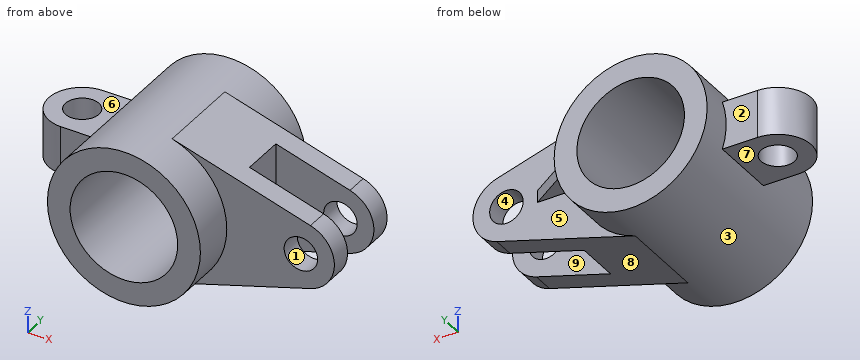
from build123d import *

# Parameters (mm, degrees)
SKETCH_1_R               = 32
SKETCH_1_R_2             = 22.5
EXTRUDE_1_DEPTH          = 72
SKETCH_2_R               = 7
EXTRUDE_2_DEPTH          = 36
CUT_EXTRUDE_1_DEPTH      = 9
EXTRUDE_3_DEPTH          = 14
SKETCH_5_R               = 7
CUT_EXTRUDE_2_DEPTH      = 33
CUT_EXTRUDE_2_DEPTH_BACK = 33
CUT_EXTRUDE_3_DEPTH      = 23
CUT_EXTRUDE_3_DEPTH_BACK = 43
EXTRUDE_4_DEPTH          = 2.5


with BuildPart() as part:
    # 草图1 → 凸台-拉伸1 (new body)
    with BuildSketch(Plane(origin=(0, 0, 0), x_dir=(1, 0, 0), z_dir=(0, 1, 0))):
        Circle(SKETCH_1_R)
        Circle(SKETCH_1_R_2, mode=Mode.SUBTRACT)
    extrude(amount=EXTRUDE_1_DEPTH)

    # 草图2 → 凸台-拉伸2 (add)
    with BuildSketch(Plane(origin=(0, 18, 0), x_dir=(1, 0, 0), z_dir=(0, 1, 0))):
        with BuildLine():
            Line((9.142857143, 30.66607512), (67, 13.416407865))
            ThreePointArc((67, 13.416407865), (77, 0), (67, -13.416407865))
            Line((67, -13.416407865), (9.142857143, -30.66607512))
            ThreePointArc((9.142857143, -30.66607512), (32, 0), (9.142857143, 30.66607512))
        make_face()
        with Locations((63, 0)):
            Circle(SKETCH_2_R, mode=Mode.SUBTRACT)
    extrude(amount=EXTRUDE_2_DEPTH)

    # 草图3 → 切除-拉伸1 (cut, symmetric)
    with BuildSketch(Plane(origin=(0, 36, 0), x_dir=(1, 0, 0), z_dir=(0, 1, 0))):
        with BuildLine():
            Line((36, 22.658822172), (36, -22.658822172))
            Line((36, -22.658822172), (67, -13.416407865))
            ThreePointArc((67, -13.416407865), (77, 0), (67, 13.416407865))
            Line((67, 13.416407865), (36, 22.658822172))
        make_face()
    extrude(amount=CUT_EXTRUDE_1_DEPTH, both=True, mode=Mode.SUBTRACT)

    # 草图4 → 凸台-拉伸3 (add, symmetric)
    with BuildSketch(Plane(origin=(0, 45, 0), x_dir=(1, 0, 0), z_dir=(0, 1, 0))):
        with BuildLine():
            Line((-30.330505487, 10), (-45, 10))
            Line((-45, 10), (-59, 10))
            Line((-59, 10), (-59, -10))
            Line((-59, -10), (-45, -10))
            Line((-45, -10), (-30.330505487, -10))
            ThreePointArc((-30.330505487, -10), (-31.936492655, 0), (-30.330505487, 10))
        make_face()
    extrude(amount=EXTRUDE_3_DEPTH, both=True)

    # 草图5 → 切除-拉伸2 (cut, two sides)
    with BuildSketch(Plane.XY) as cut_extrude_2_sk:
        with Locations((-45, 45)):
            Circle(SKETCH_5_R)
    extrude(amount=CUT_EXTRUDE_2_DEPTH, mode=Mode.SUBTRACT)
    extrude(cut_extrude_2_sk.sketch, amount=-CUT_EXTRUDE_2_DEPTH_BACK, mode=Mode.SUBTRACT)

    # 草图6 → 切除-拉伸3 (cut, two sides)
    with BuildSketch(Plane.XY.offset(10)) as cut_extrude_3_sk:
        with BuildLine():
            Line((-45, 59), (-45, 73.390549991))
            Line((-45, 73.390549991), (-74.161740497, 70.167226716))
            Line((-74.161740497, 70.167226716), (-67.715093947, 21.172712935))
            Line((-67.715093947, 21.172712935), (-45.42483437, 31.00644735))
            ThreePointArc((-45.42483437, 31.00644735), (-58.99838807, 45.212441645), (-45, 59))
        make_face()
    extrude(amount=CUT_EXTRUDE_3_DEPTH, mode=Mode.SUBTRACT)
    extrude(cut_extrude_3_sk.sketch, amount=-CUT_EXTRUDE_3_DEPTH_BACK, mode=Mode.SUBTRACT)

    # 草图7 → 凸台-拉伸4 (add, symmetric)
    with BuildSketch(Plane.XY):
        Polygon((50, 54), (28.987302247, 67.645805474), (28.987302247, 54), align=None)
    extrude(amount=EXTRUDE_4_DEPTH, both=True)


solid = part.part
The listing builds one solid part. Answer for the finished solid, in the listing's coordinates (mm). Face numbers are marked on the shaded views. A direction names the side the tool comes from. Give positions to 0.01 mm unless a question says otherwise; leave off trailing zeros. Write each loop counter-clockwise with the first axis right and the second up, starting at its lowest first coordinate (ties: lowest second). Pieces come first, ordered by that corner, then holes.
1) Section B-B (y = 41) is taken. Write down the section's boundary in (x, z).
2) Section A-A (x = 0) is taken. Write down the section's boundary in (y, z).
3) For a pull along Z with two mould halves and no side action, classify the marked faces 1, 2, 3 and 4 as pulls with the +Z half, pulls with the -Z half, needs draft (parallel to the pull), parting line crosses it, or undercut.
4) A tool of negligible diameter and unlimited length cuts with its end or side. For the marked faces 5, 6, 7, 8 and 9, from which of +Z, -Z, +X, -X, +Y, -Y can it reach the whole face along a straight path? Write none if from no direction.
5) Section D-D (z = -15) is taken. Write down the section's boundary in (x, y).
6) Find the intervals of material crossed by L1, parallel to X at y = 29, z = 0; L2, parallel to X at y = 47.25, z = 0; L3, parallel to Y at x = -45, z = 5, in increasing order.
7) Section C-C (z = 0) is taken. Count the separate pieces of the cut face and the enclosed holes in it, and give its area (3 significant figures).
8) Given P1, Ø1, axis at y = 29.5, z = -17, coming from the +X side; P2, Ø1, axis at x = 39.5, y = 46, coming from the +Z side; P3, Ø12, axis at x = -20, y = 44, coming from the +Z side (3 decimals), each flat-ended and moving along its own axis, determine where each tip first touches the part or whether it passes through.
Response:
1. outline: (-58.42, -10) - (-50.74, -10) - (-50.74, 10) - (-58.42, 10) - close; (-39.26, -10) - (-30.4, -10) arc R32 ccw to (9.14, -30.67) - (36, -22.66) - (36, 22.66) - (9.14, 30.67) arc R32 ccw to (-30.4, 10) - (-39.26, 10) - close; hole circle Ø45 at (0, 0)
2. outline: (0, -32) - (72, -32) - (72, -22.5) - (0, -22.5) - close; (0, 22.5) - (72, 22.5) - (72, 32) - (0, 32) - close
3. face 1: undercut
3. face 2: needs draft
3. face 3: parting line crosses it
3. face 4: undercut
4. face 5: +X, +Y
4. face 6: +Z, -X, +Y, -Y
4. face 7: -Z, -X, +Y, -Y
4. face 8: -Z, +X, +Y, -Y
4. face 9: +Z, -Z, +X
5. outline: (-28.27, 0) - (-16.77, 0) - (-16.77, 72) - (-28.27, 72) - close; (16.77, 0) - (28.27, 0) - (28.27, 18) - (61.69, 18) - (61.69, 27) - (36, 27) - (36, 45) - (61.69, 45) - (61.69, 54) - (28.27, 54) - (28.27, 72) - (16.77, 72) - close
6. L1: x = -32 to -22.5, 22.5 to 36
6. L2: x = -58.82 to -51.63, -38.37 to -22.5, 22.5 to 56, 70 to 77
6. L3: y = 31 to 38, 52 to 59
7. separate pieces: 4
7. enclosed holes: 1
7. area: 2,620 mm2
8. P1: stops at x = 36
8. P2: stops at z = 21.76
8. P3: stops at z = 28.775
